```python
from build123d import *

# Parameters (mm, degrees)
SKETCH_1_W          = 20
SKETCH_1_H          = 40
SKETCH_1_W_2        = 18
SKETCH_1_H_2        = 38
EXTRUDE_1_DEPTH     = 240
SKETCH_2_R          = 1.6
CUT_EXTRUDE_1_DEPTH = 245.131112315
SKETCH_3_R          = 1.6
SKETCH_3_R_2        = 1.599999999
CUT_EXTRUDE_2_DEPTH = 245.131112315
SKETCH_4_R          = 14.5
CUT_EXTRUDE_3_DEPTH = 245.131112315


with BuildPart() as part:
    # 草图1 → 凸台-拉伸1 (new body)
    with BuildSketch(Plane.XY):
        with Locations((10, 20)):
            Rectangle(SKETCH_1_W, SKETCH_1_H)
        with Locations((10, 20)):
            Rectangle(SKETCH_1_W_2, SKETCH_1_H_2, mode=Mode.SUBTRACT)
    extrude(amount=EXTRUDE_1_DEPTH)

    # 草图2 → 切除-拉伸1 (cut, through all)
    with BuildSketch(Plane(origin=(20, 0, 0), x_dir=(0, 0, -1), z_dir=(1, 0, 0))):
        with Locations((-10, 8)):
            Circle(SKETCH_2_R)
        with Locations((-34, 8)):
            Circle(SKETCH_2_R)
        with Locations((-84, 4.000000001)):
            Circle(SKETCH_2_R)
        with Locations((-94, 4.000000001)):
            Circle(SKETCH_2_R)
        with Locations((-108, 16.000000001)):
            Circle(SKETCH_2_R)
        with Locations((-118, 16.000000001)):
            Circle(SKETCH_2_R)
        with Locations((-108, 4.000000001)):
            Circle(SKETCH_2_R)
        with Locations((-118, 4.000000001)):
            Circle(SKETCH_2_R)
        with Locations((-84, 16.000000001)):
            Circle(SKETCH_2_R)
        with Locations((-94, 16.000000001)):
            Circle(SKETCH_2_R)
        with Locations((-10, 32)):
            Circle(SKETCH_2_R)
        with Locations((-34, 32)):
            Circle(SKETCH_2_R)
        with Locations((-22, 32)):
            Circle(SKETCH_2_R)
        with Locations((-22, 8)):
            Circle(SKETCH_2_R)
    extrude(amount=-CUT_EXTRUDE_1_DEPTH, mode=Mode.SUBTRACT)

    # 草图3 → 切除-拉伸2 (cut, through all)
    with BuildSketch(Plane(origin=(0, 40, 0), x_dir=(1, 0, 0), z_dir=(0, 1, 0))):
        with Locations(Location((6, -227.5, 0), (0, 0, 270))):
            Circle(SKETCH_3_R)
        with Locations(Location((14, -227.5, 0), (0, 0, 270))):
            Circle(SKETCH_3_R)
        with Locations(Location((16.000000001, -191.000000001, 0), (0, 0, 270))):
            Circle(SKETCH_3_R_2)
        with Locations(Location((16.000000001, -181.000000001, 0), (0, 0, 270))):
            Circle(SKETCH_3_R_2)
        with Locations(Location((4.000000001, -167.000000001, 0), (0, 0, 270))):
            Circle(SKETCH_3_R_2)
        with Locations(Location((4.000000001, -157.000000001, 0), (0, 0, 270))):
            Circle(SKETCH_3_R_2)
        with Locations(Location((16.000000001, -167.000000001, 0), (0, 0, 270))):
            Circle(SKETCH_3_R_2)
        with Locations(Location((16.000000001, -157.000000001, 0), (0, 0, 270))):
            Circle(SKETCH_3_R_2)
        with Locations(Location((4.000000001, -191.000000001, 0), (0, 0, 270))):
            Circle(SKETCH_3_R_2)
        with Locations(Location((4.000000001, -181.000000001, 0), (0, 0, 270))):
            Circle(SKETCH_3_R_2)
        with Locations(Location((6, -220, 0), (0, 0, 270))):
            Circle(SKETCH_3_R)
        with Locations(Location((14, -220, 0), (0, 0, 270))):
            Circle(SKETCH_3_R)
        with Locations(Location((6, -235, 0), (0, 0, 270))):
            Circle(SKETCH_3_R)
        with Locations(Location((14, -235, 0), (0, 0, 270))):
            Circle(SKETCH_3_R)
    extrude(amount=-CUT_EXTRUDE_2_DEPTH, mode=Mode.SUBTRACT)

    # 草图4 → 切除-拉伸3 (cut, through all)
    with BuildSketch(Plane(origin=(20, 0, 0), x_dir=(0, 0, -1), z_dir=(1, 0, 0))):
        with Locations((-220, 20)):
            Circle(SKETCH_4_R)
        with Locations((-180, 20)):
            Circle(SKETCH_4_R)
        with Locations((-140, 20)):
            Circle(SKETCH_4_R)
        with Locations((-60, 20)):
            Circle(SKETCH_4_R)
    extrude(amount=-CUT_EXTRUDE_3_DEPTH, mode=Mode.SUBTRACT)


solid = part.part
```
The listing builds one solid part. Answer for the finished solid, in the listing's coordinates (mm). A direction names the side the tool comes from. Round coordinates to 2 decimals unless told otherwise and drop trailing zeros. Loops run counter-clockwise (first coordinate to the right, second up) from the corner with the lowest first, then second, coordinate; pieces in that order, holes last.
1) A cutting plane is placed at C-C on y = 20. Give the number of separate pieces and of enclosed holes in the cut face, plus the area to 3 significant figures.
Outcome:
separate pieces: 10
enclosed holes: 0
area: 248 mm2
2) For faces 1 (the face through (10, 39, 118)), 2 (the face through (19.507, 20.638, 74.486)), determine the directions among +Z, -Z, +X, -X, +Y, -Y from which every point of the face is accessible in a straight line to the end or side of a thin tool.
Outcome:
face 1: +Z, -Z
face 2: +X, -X
3) A cutting plane is placed at B-B on z = 76.5. Determine the outline of the cut face in (x, y).
Outcome:
outline: (0, 0) - (20, 0) - (20, 40) - (0, 40) - close; hole (1, 1) - (19, 1) - (19, 39) - (1, 39) - close
4) Consider line 1 (Y direction, x = 0.7, z = 84); line 2 (X direction, y = 25, z = 74.5); line 3 (Y direction, x = 19.3, z = 180). Determine where each line is inside the solid, lowest interval first.
Outcome:
line 1: y = 0 to 2.4, 5.6 to 14.4, 17.6 to 40
line 2: x = 0 to 1, 19 to 20
line 3: y = 0 to 5.5, 34.5 to 40
5) For a pull along X with two mould halves and no side action, classify faces 3 (the face through (0, 20, 92)), 4 (the face through (19, 20, 92)), 5 (the face through (10, 0, 118)) as released by +X, released by -X, zero draft, split by the parting line, or undercut.
Outcome:
face 3: released by -X
face 4: undercut
face 5: zero draft
6) A cutting plane is placed at A-A on z = 48.5. Determine the outline of the cut face in (x, y).
Outcome:
outline: (0, 0) - (20, 0) - (20, 11.17) - (19, 11.17) - (19, 1) - (1, 1) - (1, 11.17) - (0, 11.17) - close; (0, 28.83) - (1, 28.83) - (1, 39) - (19, 39) - (19, 28.83) - (20, 28.83) - (20, 40) - (0, 40) - close
